Model file for the job. Use its own axes, mm. A direction names the side the tool comes from. Give positions to 0.01 mm unless a question says otherwise; leave off trailing zeros. Write each loop counter-clockwise with the first axis right and the second up, starting at its lowest first coordinate (ties: lowest second). Pieces come first, ordered by that corner, then holes.
```python
from build123d import *

# Parameters (mm, degrees)
BOSS_EXTRUDE1_DEPTH      = 25.4
BOSS_EXTRUDE1_DEPTH_BACK = 406.4
SKETCH2_R                = 12.7
CUT_EXTRUDE1_DEPTH       = 25.4
SKETCH3_R                = 2.4892
CUT_EXTRUDE2_DEPTH       = 1
CUT_EXTRUDE2_DEPTH_BACK  = 51.8


with BuildPart() as part:
    # Sketch1 → Boss-Extrude1 (new body, two sides)
    with BuildSketch(Plane(origin=(0, 0, 0), x_dir=(-1, 0, 0), z_dir=(0, 0, -1))) as boss_extrude1_sk:
        with BuildLine():
            Line((-12.7, 25.146), (-12.7, -25.146))
            ThreePointArc((-12.7, -25.146), (-12.625605122, -25.325605122), (-12.446, -25.4))
            Line((-12.446, -25.4), (12.446, -25.4))
            ThreePointArc((12.446, -25.4), (12.625605122, -25.325605122), (12.7, -25.146))
            Line((12.7, -25.146), (12.7, 25.146))
            ThreePointArc((12.7, 25.146), (12.625605122, 25.325605122), (12.446, 25.4))
            Line((12.446, 25.4), (-12.446, 25.4))
            ThreePointArc((-12.446, 25.4), (-12.625605122, 25.325605122), (-12.7, 25.146))
        make_face()
        with BuildLine():
            Line((-11.1125, -22.225), (-11.1125, 22.225))
            ThreePointArc((-11.1125, 22.225), (-10.647532015, 23.347532015), (-9.525, 23.8125))
            Line((-9.525, 23.8125), (9.525, 23.8125))
            ThreePointArc((9.525, 23.8125), (10.647532015, 23.347532015), (11.1125, 22.225))
            Line((11.1125, 22.225), (11.1125, -22.225))
            ThreePointArc((11.1125, -22.225), (10.647532015, -23.347532015), (9.525, -23.8125))
            Line((9.525, -23.8125), (-9.525, -23.8125))
            ThreePointArc((-9.525, -23.8125), (-10.647532015, -23.347532015), (-11.1125, -22.225))
        make_face(mode=Mode.SUBTRACT)
    extrude(amount=BOSS_EXTRUDE1_DEPTH)
    extrude(boss_extrude1_sk.sketch, amount=-BOSS_EXTRUDE1_DEPTH_BACK)

    # Sketch2 → Cut-Extrude1 (cut)
    with BuildSketch(Plane.ZY.offset(12.7)):
        with Locations((19.05, 1.778)):
            Circle(SKETCH2_R)
    extrude(amount=-CUT_EXTRUDE1_DEPTH, mode=Mode.SUBTRACT)

    # Sketch3 → Cut-Extrude2 (cut, two sides)
    with BuildSketch(Plane.XZ.offset(25.4)) as cut_extrude2_sk:
        with Locations((0, 50.8)):
            Circle(SKETCH3_R)
        with Locations((0, 71.581818182)):
            Circle(SKETCH3_R)
        with Locations((0, 92.363636364)):
            Circle(SKETCH3_R)
        with Locations((0, 113.145454545)):
            Circle(SKETCH3_R)
        with Locations((0, 133.927272727)):
            Circle(SKETCH3_R)
        with Locations((0, 154.709090909)):
            Circle(SKETCH3_R)
        with Locations((0, 175.490909091)):
            Circle(SKETCH3_R)
        with Locations((0, 196.272727273)):
            Circle(SKETCH3_R)
        with Locations((0, 217.054545455)):
            Circle(SKETCH3_R)
        with Locations((0, 237.836363636)):
            Circle(SKETCH3_R)
        with Locations((0, 258.618181818)):
            Circle(SKETCH3_R)
        with Locations((0, 342.9)):
            Circle(SKETCH3_R)
        with Locations((0, 279.4)):
            Circle(SKETCH3_R)
    extrude(amount=CUT_EXTRUDE2_DEPTH, mode=Mode.SUBTRACT)
    extrude(cut_extrude2_sk.sketch, amount=-CUT_EXTRUDE2_DEPTH_BACK, mode=Mode.SUBTRACT)


solid = part.part
```
1. Probe probe 1 along Y at (x, z) = (-12.3, 19.05); probe 2 along X at (y, z) = (1, 303.5); probe 3 along Y at (x, z) = (-3.75, 91). List the from-to ranges inside material, lowest first.
Calculated:
probe 1: y = -25.4 to -10.92, 14.48 to 25.4
probe 2: x = -12.7 to -11.11, 11.11 to 12.7
probe 3: y = -25.4 to -23.81, 23.81 to 25.4
2. Slice it at B-B, the plane y = -7. Write the cut outline in (x, z).
Calculated:
outline: (-12.7, -25.4) - (-11.11, -25.4) - (-11.11, 9.87) - (-12.7, 9.87) - close; (-12.7, 28.23) - (-11.11, 28.23) - (-11.11, 406.4) - (-12.7, 406.4) - close; (11.11, -25.4) - (12.7, -25.4) - (12.7, 9.87) - (11.11, 9.87) - close; (11.11, 28.23) - (12.7, 28.23) - (12.7, 406.4) - (11.11, 406.4) - close
3. Which spindle directions (+Z, -Z, +X, -X, +Y, -Y) get a long thin tool onto all of the face, cutting with end or side? Do faces 1 (the flat face through (0, 23.812, 187)), 2 (the flat face through (11.3, 2, -25.4)). Say none if no direction does.
Calculated:
face 1: +Z, -Z
face 2: -Z, +X, -X, +Y, -Y
4. Pull direction Y, two halves, no side cores. Call faces 3 (the flat face through (-12.7, 0, 187)), 4 (the flat face through (11.112, 0, 187)), 5 (the flat face through (0, -25.4, 187)), 6 (the flat face through (-11.112, 0, 187)): +Y half, -Y half, draft (parallel to the pull), parting line (faces both ways), or undercut.
Calculated:
face 3: draft
face 4: undercut
face 5: -Y half
face 6: undercut
